Geometry check sheet. Reference: the model listing, model coordinates, mm. Face numbers are marked on the shaded views. A direction names the side the tool comes from. Coordinates: 2 decimals unless noted, no trailing zeros. Order: outer loops, then holes, each group sorted by start corner. A loop starts at its lowest first (then second) coordinate and runs counter-clockwise, first axis right, second up. Notation, with made-up numbers: (-0.75, 33) - (51.25, 33) arc R23 cw to (51.25, 53) - close; hole circle Ø2 at (-10, 3.25). An arc over 180 degrees is marked (long way). Put each result on its own line as item: value.
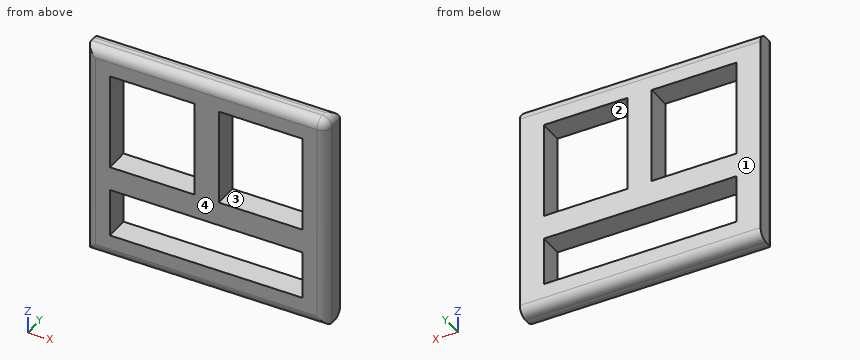
from build123d import *

# Parameters (mm, degrees)
F0_W     = 12.7
F0_H     = 50.8
F1_DEPTH = 12.7
F2_R     = 5.08


with BuildPart() as f1:
    # F0 (on Front) → F1 (new body)
    with BuildSketch(Plane.XZ):
        Polygon((-63.5, 25.4), (-63.5, -25.4), (63.5, -25.4), (63.5, 25.4), (63.5, 88.9), (-63.5, 88.9), align=None)
        Polygon((-50.8, 12.7), (-50.8, 25.4), (-50.8, 76.2), (-6.031548, 76.2), (6.668452, 76.2), (50.8, 76.2), (50.8, 25.4), (50.8, 12.7), (50.8, -12.7), (-50.8, -12.7), align=None, mode=Mode.SUBTRACT)
        Polygon((-6.031548, 25.4), (-50.8, 25.4), (-50.8, 12.7), (50.8, 12.7), (50.8, 25.4), (6.668452, 25.4), align=None)
        with Locations((0.318452, 50.8)):
            Rectangle(F0_W, F0_H)
    extrude(amount=F1_DEPTH)

    # F2
    f2_edges = [f1.edges().sort_by_distance(p)[0] for p in [
        (0, 0, 88.9),
        (0, 0, -25.4),
        (63.5, -12.7, 31.75),
        (63.5, -6.35, 88.9),
        (0, -12.7, 88.9),
        (-63.5, -12.7, 31.75),
        (0, -12.7, -25.4),
    ]]
    fillet(f2_edges, radius=F2_R)


solid = f1.part
Q1. Section check D-D on y = -9.5. Record the boundary of the cut face in (x, z), then the cut area to 3 significant figures.
Answer block:
outline: (-63.14, -25.04) - (63.14, -25.04) - (63.14, 83.82) arc R4.72 ccw to (58.42, 88.54) - (-63.14, 88.54) - close; hole (-50.8, -12.7) - (50.8, -12.7) - (50.8, 12.7) - (-50.8, 12.7) - close; hole (-50.8, 25.4) - (-6.03, 25.4) - (-6.03, 76.2) - (-50.8, 76.2) - close; hole (6.67, 25.4) - (50.8, 25.4) - (50.8, 76.2) - (6.67, 76.2) - close
area: 7,240 mm^2
Q2. Section check B-B on z = 47. Record the boundary of the cut face in (x, y), then the cut area to 3 significant figures.
Answer block:
outline: (-63.5, -7.62) arc R5.08 ccw to (-58.42, -12.7) - (-50.8, -12.7) - (-50.8, 0) - (-63.5, 0) - close; (-6.03, -12.7) - (6.67, -12.7) - (6.67, 0) - (-6.03, 0) - close; (50.8, -12.7) - (58.42, -12.7) arc R5.08 ccw to (63.5, -7.62) - (63.5, 0) - (50.8, 0) - close
area: 473 mm^2
Q3. Depth check by flat-ended pin: pin 1 Ø1 at (y, z) = (-9.5, 41) entering from +X; pin 2 Ø5 at (x, y) = (-46, -2) entering from -Z. Enter the tip coordinate at first touch or a pass-through.
Answer block:
pin 1: stops at x = 63.31
pin 2: stops at z = -25.37
Q4. Draft check along X on the marked faces 3 and 4. Enter one of: pulls with the +X half, pulls with the -X half, needs draft (parallel to the pull), parting line crosses it, or undercut.
Answer block:
face 3: undercut
face 4: needs draft
Q5. Thickness scan on L1, parallel to X at y = -6.75, z = 46.5; L2, parallel to Z at x = 34.5, y = -5.25; L3, parallel to Z at x = 2, y = -4.5. Record the ranges inside material, lowest first. Write a range as [from, to].
Answer block:
L1: x = [-63.5, -50.8], [-6.03, 6.67], [50.8, 63.5]
L2: z = [-25.4, -12.7], [12.7, 25.4], [76.2, 88.9]
L3: z = [-25.37, -12.7], [12.7, 88.87]
Q6. Section check C-C on z = -10. Record the boundary of the cut face in (x, y).
Answer block:
outline: (-63.5, -7.62) arc R5.08 ccw to (-58.42, -12.7) - (-50.8, -12.7) - (-50.8, 0) - (-63.5, 0) - close; (50.8, -12.7) - (58.42, -12.7) arc R5.08 ccw to (63.5, -7.62) - (63.5, 0) - (50.8, 0) - close
Q7. Section check A-A on x = 19.5. Record the boundary of the cut face in (y, z), then the cut area to 3 significant figures.
Answer block:
outline: (-12.7, -20.32) arc R5.08 ccw to (-7.62, -25.4) - (-5.08, -25.4) arc R5.08 ccw to (0, -20.32) - (0, -12.7) - (-12.7, -12.7) - close; (-12.7, 12.7) - (0, 12.7) - (0, 25.4) - (-12.7, 25.4) - close; (-12.7, 76.2) - (0, 76.2) - (0, 83.82) arc R5.08 ccw to (-5.08, 88.9) - (-7.62, 88.9) arc R5.08 ccw to (-12.7, 83.82) - close
area: 462 mm^2
Q8. Access from +Z, -Z, +X, -X, +Y, -Y to the whole of each face (thin tool, end or side, straight path). Record for the marked faces 1 and 2.
Answer block:
face 1: +Z, -Z, +X, -X, +Y
face 2: +Y, -Y
